Answer from the drawing. Dimensions are ordinates in mm from the lowest x, y and z of the part. A direction names the side the tool comes from. Give positions to 0.01 mm unless a question says otherwise; leave off trailing zeros. Loops run counter-clockwise (first coordinate to the right, second up) from the corner with the lowest first, then second, coordinate; pieces in that order, holes last. Notation, with made-up numbers: M 80.25,14 L 135.25,14 A22 cw 135.25,44 Z; hole C 61,6.5 d6. An arc over 180 degrees is marked long. Return JSON: item names as keys, results as strings. Group by question number.
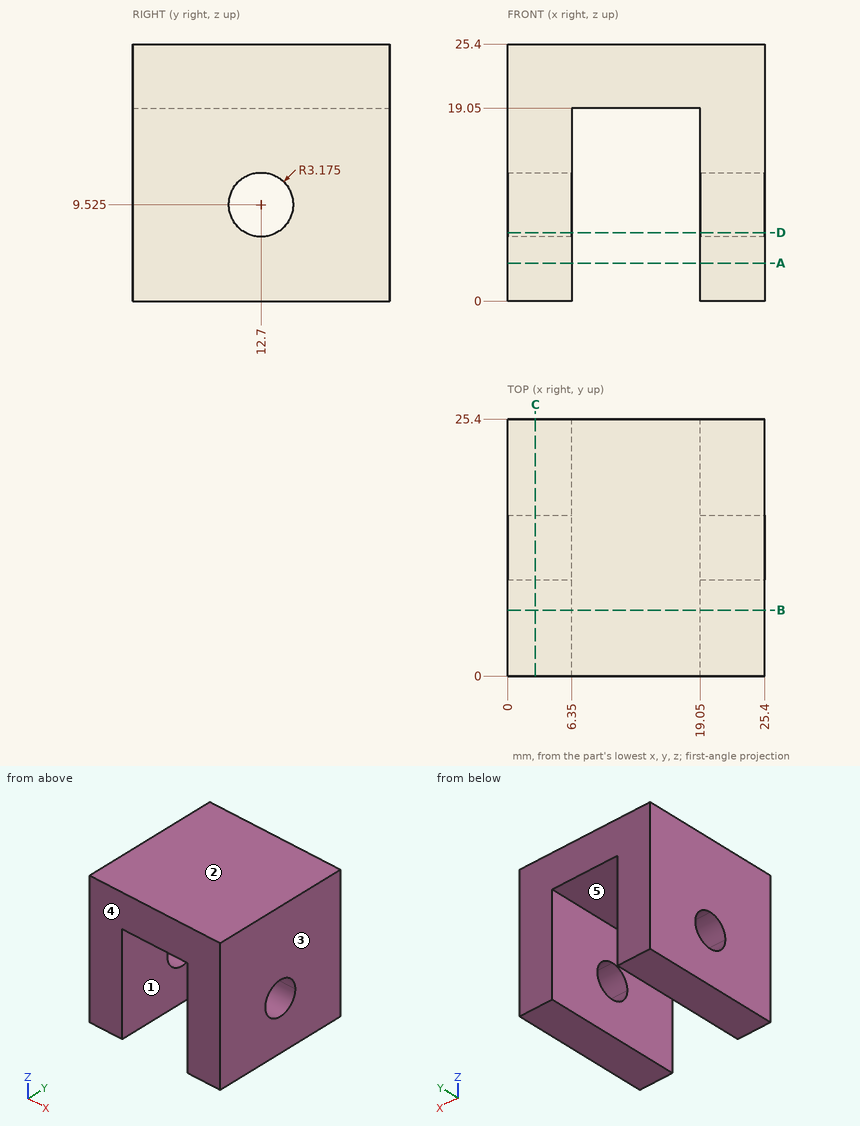
1. Find section C-C (x = 2.75). Write down the section's boundary in (y, z) (3 decimals), and give its area (3 significant figures).
2. The mould has two halves that part along X. Classify the marked faces 3, 4 and 5: +X half, -X half, draft (parallel to the pull), parting line (faces both ways), or undercut.
3. Find section A-A (z = 3.75). Write down the section's boundary in (x, y).
4. Straight lines are drawn through the part: line 1 along X through (y, z) = (24, 7.25); line 2 along Y through (x, z) = (19.25, 9.5); line 3 along Z through (x, y) = (9.75, 6.75). For each, find the intervals that lie inside material, in ascending order.
5. Find section B-B (y = 6.5). Write down the section's boundary in (x, z).
6. For the marked faces 1 and 2, determine the directions among +Z, -Z, +X, -X, +Y, -Y from which every point of the face is accessible in a straight line to the end or side of a thin tool.
7. Find section D-D (z = 6.75). Write down the section's boundary in (x, y), and give its area (3 significant figures).
8. Flat-ended cylindrical pins translate along their axes: P1, Ø5, axis at x = 9, z = 8.5, coming from the -Y side; P2, Ø4, axis at x = 11.5, y = 12.5, coming from the -Z side. Find the tip coordinate at first contact, or state that the pin passes through.
Result:
{
 "1": {"outline": "M 0,0 L 25.4,0 L 25.4,25.4 L 0,25.4 Z; hole C 12.7,9.525 d6.35", "area": "613 mm2"},
 "2": {"face 3": "+X half", "face 4": "draft", "face 5": "undercut"},
 "3": {"outline": "M 0,0 L 6.35,0 L 6.35,25.4 L 0,25.4 Z; M 19.05,0 L 25.4,0 L 25.4,25.4 L 19.05,25.4 Z"},
 "4": {"line 1": "x = 0 to 6.35, 19.05 to 25.4", "line 2": "y = 0 to 9.53, 15.87 to 25.4", "line 3": "z = 19.05 to 25.4"},
 "5": {"outline": "M 0,0 L 6.35,0 L 6.35,19.05 L 19.05,19.05 L 19.05,0 L 25.4,0 L 25.4,25.4 L 0,25.4 Z"},
 "6": {"face 1": "-Z, +Y, -Y", "face 2": "+Z, +X, -X, +Y, -Y"},
 "7": {"outline": "M 0,0 L 6.35,0 L 6.35,11.16 L 0,11.16 Z; M 0,14.24 L 6.35,14.24 L 6.35,25.4 L 0,25.4 Z; M 19.05,0 L 25.4,0 L 25.4,11.16 L 19.05,11.16 Z; M 19.05,14.24 L 25.4,14.24 L 25.4,25.4 L 19.05,25.4 Z", "area": "283 mm2"},
 "8": {"P1": "passes through", "P2": "stops at z = 19.05"}
}
